The model under review builds one solid part; all positions refer to its coordinate system, in mm. A direction names the side the tool comes from. Round coordinates to 2 decimals unless told otherwise and drop trailing zeros. Order: outer loops, then holes, each group sorted by start corner. A loop starts at its lowest first (then second) coordinate and runs counter-clockwise, first axis right, second up. Notation, with made-up numbers: (24, 56.25) -> (51, 56.25) arc R24 ccw to (51, 81.25) -> close; hole circle Ø11 at (-20, 0.25). An arc over 180 degrees is marked (long way). Use a Markdown table: item, result. Add a question column.
```python
from build123d import *

# Parameters (mm, degrees)
SKETCH1_R                    = 1.625
BOSS_EXTRUDE1_DEPTH          = 2.5
FILLET1_R                    = 5
FILLET2_R                    = 5
CHAMFER2_SIZE                = 1.6
SKETCH2_W                    = 10
SKETCH2_H                    = 10
BOSS_EXTRUDE2_DEPTH          = 10
SKETCH3_R                    = 1.6
CUT_EXTRUDE1_DEPTH           = 3.2
SKETCH4_R                    = 1.6
CUT_EXTRUDE2_DEPTH           = 3.2
CHAMFER1_SIZE                = 6
BOSS_EXTRUDE3_DEPTH          = 5
CIRPATTERN1_COUNT            = 4
CHAMFER1_OF_CIRPATTERN1_SIZE = 6
SKETCH7_R                    = 5
CUT_EXTRUDE5_DEPTH           = 2.5
SKETCH6_R                    = 5
CUT_EXTRUDE6_DEPTH           = 2.5
CUT_EXTRUDE7_START           = -2.5
SKETCH8_R                    = 5
CUT_EXTRUDE7_DEPTH           = 2.5
CUT_EXTRUDE8_START           = -2.5
SKETCH9_R                    = 5
CUT_EXTRUDE8_DEPTH           = 2.5


with BuildPart() as part:
    # Sketch1 → Boss-Extrude1 (new body)
    with BuildSketch(Plane(origin=(0, 0, 0), x_dir=(1, 0, 0), z_dir=(0, 1, 0))):
        Polygon((-52.5, 45), (-52.5, -45), (-52.5, -52.5), (-45, -52.5), (-45, -50), (-42.127158908, -50), (-6, -4), (6, -4), (42.127158908, -50), (45, -50), (45, -52.5), (52.5, -52.5), (52.5, -45), (52.5, 45), (52.5, 52.5), (45, 52.5), (45, 50), (42.127158908, 50), (6, 4), (-6, 4), (-42.127158908, 50), (-45, 50), (-45, 52.5), (-52.5, 52.5), align=None)
        with Locations(Location((-45, 45, 0), (0, 0, 270))):
            Circle(SKETCH1_R, mode=Mode.SUBTRACT)
        with Locations(Location((45, 45, 0), (0, 0, 270))):
            Circle(SKETCH1_R, mode=Mode.SUBTRACT)
        with Locations(Location((45, -45, 0), (0, 0, 270))):
            Circle(SKETCH1_R, mode=Mode.SUBTRACT)
        with Locations(Location((-45, -45, 0), (0, 0, 270))):
            Circle(SKETCH1_R, mode=Mode.SUBTRACT)
        Polygon((-50, 40), (-50, -40), (-38.088044946, -40), (-6.673124156, 0), (-38.088044946, 40), align=None, mode=Mode.SUBTRACT)
        Polygon((50, -40), (38.088044946, -40), (6.673124156, 0), (38.088044946, 40), (50, 40), align=None, mode=Mode.SUBTRACT)
    extrude(amount=BOSS_EXTRUDE1_DEPTH)

    # Fillet1
    fillet1_edges = [part.edges().sort_by_distance(p)[0] for p in [
        (6, 1.25, 4),
        (-6, 1.25, 4),
        (-6, 1.25, -4),
        (6, 1.25, -4),
        (-6.673124156, 1.25, 0),
        (6.673124156, 1.25, 0),
    ]]
    fillet(fillet1_edges, radius=FILLET1_R)

    # Fillet2
    fillet2_edges = [part.edges().sort_by_distance(p)[0] for p in [
        (-38.088044946, 1.25, -40),
        (-50, 1.25, -40),
        (-50, 1.25, 40),
        (-38.088044946, 1.25, 40),
        (50, 1.25, 40),
        (50, 1.25, -40),
        (38.088044946, 1.25, -40),
        (38.088044946, 1.25, 40),
    ]]
    fillet(fillet2_edges, radius=FILLET2_R)

    # Chamfer2
    chamfer2_edges = [part.edges().sort_by_distance(p)[0] for p in [
        (-45, 0, -46.625),
        (45, 0, -46.625),
        (45, 0, 43.375),
        (-45, 0, 43.375),
    ]]
    chamfer(chamfer2_edges, length=CHAMFER2_SIZE)

    # Sketch2 → Boss-Extrude2 (add)
    with BuildSketch(Plane(origin=(0, 2.5, 0), x_dir=(1, 0, 0), z_dir=(0, 1, 0))):
        with Locations((-45, 45)):
            Rectangle(SKETCH2_W, SKETCH2_H)
    boss_extrude2 = extrude(amount=BOSS_EXTRUDE2_DEPTH)

    # Sketch3 → Cut-Extrude1 (cut)
    with BuildSketch(Plane.ZY.offset(50)):
        with Locations((-45, 7.5)):
            Circle(SKETCH3_R)
    cut_extrude1 = extrude(amount=-CUT_EXTRUDE1_DEPTH, mode=Mode.SUBTRACT)

    # Sketch4 → Cut-Extrude2 (cut)
    with BuildSketch(Plane(origin=(0, 0, -50), x_dir=(-1, 0, 0), z_dir=(0, 0, -1))):
        with Locations((45, 7.5)):
            Circle(SKETCH4_R)
    cut_extrude2 = extrude(amount=-CUT_EXTRUDE2_DEPTH, mode=Mode.SUBTRACT)

    # Chamfer1
    chamfer1_edges = [part.edges().sort_by_distance(p)[0] for p in [
        (-40, 12.5, -45),
        (-45, 12.5, -40),
    ]]
    chamfer(chamfer1_edges, length=CHAMFER1_SIZE)

    # Sketch5 → Boss-Extrude3 (add)
    with BuildSketch(Plane(origin=(0, 2.5, 0), x_dir=(1, 0, 0), z_dir=(0, 1, 0))):
        Polygon((-45, 50), (-45, 52.5), (-52.5, 52.5), (-52.5, 45), (-50, 45), (-50, 50), align=None)
    boss_extrude3 = extrude(amount=BOSS_EXTRUDE3_DEPTH)

    # CirPattern1: Boss-Extrude2, Cut-Extrude1, Cut-Extrude2, Boss-Extrude3 ×4 about axis
    cirpattern1_axis = Axis((0, 0, 0), (0, 1, 0))
    add([boss_extrude2.rotate(cirpattern1_axis, i * 360 / CIRPATTERN1_COUNT) for i in range(1, CIRPATTERN1_COUNT)])
    add([cut_extrude1.rotate(cirpattern1_axis, i * 360 / CIRPATTERN1_COUNT) for i in range(1, CIRPATTERN1_COUNT)], mode=Mode.SUBTRACT)
    add([cut_extrude2.rotate(cirpattern1_axis, i * 360 / CIRPATTERN1_COUNT) for i in range(1, CIRPATTERN1_COUNT)], mode=Mode.SUBTRACT)
    add([boss_extrude3.rotate(cirpattern1_axis, i * 360 / CIRPATTERN1_COUNT) for i in range(1, CIRPATTERN1_COUNT)])

    # Chamfer1 of CirPattern1
    chamfer1_of_cirpattern1_edges = [part.edges().sort_by_distance(p)[0] for p in [
        (-45, 12.5, 40),
        (-40, 12.5, 45),
        (40, 12.5, 45),
        (45, 12.5, 40),
        (45, 12.5, -40),
        (40, 12.5, -45),
    ]]
    chamfer(chamfer1_of_cirpattern1_edges, length=CHAMFER1_OF_CIRPATTERN1_SIZE)

    # Sketch7 → Cut-Extrude5 (cut)
    with BuildSketch(Plane(origin=(0, 0, -52.5), x_dir=(-1, 0, 0), z_dir=(0, 0, -1))):
        with Locations((45, 7.5)):
            Circle(SKETCH7_R)
        with Locations((-45, 7.5)):
            Circle(SKETCH7_R)
    extrude(amount=-CUT_EXTRUDE5_DEPTH, mode=Mode.SUBTRACT)

    # Sketch6 → Cut-Extrude6 (cut)
    with BuildSketch(Plane.ZY.offset(52.5)):
        with Locations((-45, 7.5)):
            Circle(SKETCH6_R)
        with Locations((45, 7.5)):
            Circle(SKETCH6_R)
    extrude(amount=-CUT_EXTRUDE6_DEPTH, mode=Mode.SUBTRACT)

    # Sketch8 → Cut-Extrude7 (cut)
    with BuildSketch(Plane.XY.offset(52.5).offset(CUT_EXTRUDE7_START)):
        with Locations((-45, 7.5)):
            Circle(SKETCH8_R)
        with Locations((45, 7.5)):
            Circle(SKETCH8_R)
    extrude(amount=CUT_EXTRUDE7_DEPTH, mode=Mode.SUBTRACT)

    # Sketch9 → Cut-Extrude8 (cut)
    with BuildSketch(Plane(origin=(52.5, 0, 0), x_dir=(0, 0, -1), z_dir=(1, 0, 0)).offset(CUT_EXTRUDE8_START)):
        with Locations((-45, 7.5)):
            Circle(SKETCH9_R)
        with Locations((45, 7.5)):
            Circle(SKETCH9_R)
    extrude(amount=CUT_EXTRUDE8_DEPTH, mode=Mode.SUBTRACT)


solid = part.part
```
Q1. Add section C-C, the plane x = -5. Give the boundary of the cut face in (y, z), then the cut area to 3 significant figures.
Q2. Draft analysis for pull direction Y (two halves, no side actions). For faces 1 (the face through (-40, 4, -45)), 2 (the face through (-45, 8, -46.8)), 3 (the face through (-51.27, 4, -48.57)), state which applies: released by +Y, released by -Y, zero draft, split by the parting line, or undercut.
Q3. Add section B-B, the plane x = -22.5. Give the boundary of the cut face in (y, z), then the cut area to 3 significant figures.
Q4. To check wall thickness, follow line 1 along X through (y, z) = (7.5, -49.2); line 2 along X through (y, z) = (11.5, 45.5); line 3 along X through (y, z) = (1.8, 45) (3 decimals). State the ranges of each line that lie inside material, in increasing order.
Q5. For faces 4 (the face through (51.23, 3.93, -48.5)), 5 (the face through (-46, 6, 50)), 6 (the face through (-5.784, 1.268, 4.517)), 7 (the face through (43.414, 2.044, 44.648)), list the 3-axis set-ups (+Z, -Z, +X, -X, +Y, -Y) from which the entire face can be reached by the end or side of a thin tool; tool diameter is ignored.
Q6. For pin 1 (3.5 mm diameter, centred on y = 8, z = 44.5, fed in from +X); pin 2 (1.1 mm diameter, centred on x = 40.5, z = 49.5, fed in from -Y); pin 3 (5 mm diameter, centred on x = -45, y = 7.5, fed in from +Z); pin 4 (6 mm diameter, centred on x = 10, y = 8, fed in from -Z), all flat-tipped, find the tip position at first contact; note any pin that passes through.
Q7. Add section A-A, the plane z = -32. Give the boundary of the cut face in (x, y), then the cut area to 3 significant figures.
Return value:
| question | item | result |
|---|---|---|
| 1 | outline | (0, -4.21) -> (2.5, -4.21) -> (2.5, 4.21) -> (0, 4.21) -> close |
| 1 | area | 21.0 mm² |
| 2 | face 1 | zero draft |
| 2 | face 2 | undercut |
| 2 | face 3 | released by +Y |
| 3 | outline | (0, -25.01) -> (2.5, -25.01) -> (2.5, -20.15) -> (0, -20.15) -> close; (0, 20.15) -> (2.5, 20.15) -> (2.5, 25.01) -> (0, 25.01) -> close |
| 3 | area | 24.3 mm² |
| 4 | line 1 | -50 to -46.6, -43.4 to -41, 41 to 43.4, 46.6 to 50 |
| 4 | line 2 | -50 to -45, 45 to 50 |
| 4 | line 3 | -52.5 to -46.625, -43.375 to -38.2, 38.2 to 43.375, 46.625 to 52.5 |
| 5 | face 4 | +X, +Y |
| 5 | face 5 | +Z, +Y |
| 5 | face 6 | +Z, +Y, -Y |
| 5 | face 7 | -Y |
| 6 | pin 1 | x = 50 |
| 6 | pin 2 | y = 2.5 |
| 6 | pin 3 | z = 50 |
| 6 | pin 4 | through |
| 7 | outline | (-52.5, 0) -> (-50, 0) -> (-50, 2.5) -> (-52.5, 2.5) -> close; (-31.81, 0) -> (-27.99, 0) -> (-27.99, 2.5) -> (-31.81, 2.5) -> close; (27.99, 0) -> (31.81, 0) -> (31.81, 2.5) -> (27.99, 2.5) -> close; (50, 0) -> (52.5, 0) -> (52.5, 2.5) -> (50, 2.5) -> close |
| 7 | area | 31.6 mm² |
